Part model, mm, in its own coordinate system. Face numbers are marked on the shaded views. A direction names the side the tool comes from. Coordinates: 2 decimals unless noted, no trailing zeros. Write item = value, one per line. Start each with the question number.
Q1. Probe line 1 (Z direction, x = -103, y = -12.75); line 2 (Y direction, x = -108.5, z = -1.5). List the from-to ranges inside material, lowest first.
Q2. Pin check, flat tips, straight feed: P1, Ø6, axis at y = 6.5, z = 3.5, coming from the -X side; P2, Ø1.5, axis at x = -102.5, z = 9, coming from the +Y side; P3, Ø4, axis at x = -81, z = -5, coming from the -Y side. Stop position of each tip, or through.
Q3. Tool access for the marked faces 1, 2 and 3: list every direction of +Z, -Z, +X, -X, +Y, -Y with a clear straight run to the whole face (end or side of a thin tool).
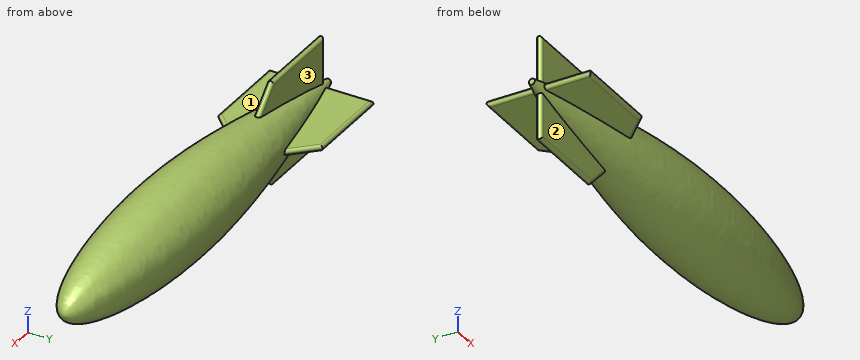
from build123d import *

# Parameters (mm, degrees)
CUT_EXTRUDE1_DEPTH      = 3.175
CUT_EXTRUDE1_DEPTH_BACK = 3.175
SKETCH3_R               = 6.509324081066561
BOSS_EXTRUDE5_DEPTH     = 0.79375
CIRPATTERN1_COUNT       = 4
FILLET2_R               = 0.79375


with BuildPart() as part:
    # Sketch2 → Revolve1 (revolve)
    with BuildSketch(Plane.XY):
        with BuildLine():
            Line((0, 0), (-127, -1.555e-14))
            add(Edge.make_bspline(
                [(-127, -1.555e-14), (-126.88600107696882, 0.01292807569490287), (-60.293650457458824, 18.501169159484686), (6.918e-14, 6.618926423252529), (0, 0)],
                knots=[0, 0, 0, 0, 0.5372544440165704, 1, 1, 1, 1], degree=3))
        make_face()
    revolve(axis=Axis((0, 0, 0), (-1, -1.2e-16, 0)))

    # Sketch3 → Cut-Extrude1 (cut, two sides: drawn at the far end of the back side and taken through both)
    with BuildSketch(Plane(origin=(-127, 0, 0), x_dir=(0, 0, -1), z_dir=(1, 0, 0)).offset(-CUT_EXTRUDE1_DEPTH_BACK)):
        Circle(SKETCH3_R)
    extrude(amount=CUT_EXTRUDE1_DEPTH + CUT_EXTRUDE1_DEPTH_BACK, mode=Mode.SUBTRACT)

    # Sketch4 → Boss-Extrude5 (add, symmetric)
    with BuildSketch(Plane.XY):
        Polygon((-120.64999999999937, 1.6175040904650868), (-120.65, 14.317504090465087), (-96.83750000000002, 14.317504090465087), (-90.2483075401766, 7.7283116306418425), (-89.68704153260985, 7.167045623074933), (-120.64999999999998, 0.8237540904650809), align=None)
    boss_extrude5 = extrude(amount=BOSS_EXTRUDE5_DEPTH, both=True)

    # CirPattern1: Boss-Extrude5 ×4 about axis
    cirpattern1_axis = Axis((0, -3.5e-16, 0), (1, 0, 0))
    for i in range(1, CIRPATTERN1_COUNT):
        add(boss_extrude5.rotate(cirpattern1_axis, i * 360 / CIRPATTERN1_COUNT))

    # Fillet2
    fillet2_edges = [part.edges().sort_by_distance(p)[0] for p in [
        (-93.52528303882053, 11.0052871292856, 0.79375),
        (-93.52528303882053, 11.005287129285604, -0.79375),
        (-108.74375, 14.317504090465087, -0.79375),
        (-108.74375, 14.317504090465087, 0.79375),
        (-120.64999999999999, 7.863429350843208, -0.79375),
        (-120.64999999999999, 7.863429350843208, 0.79375),
        (-120.64999999999999, 0.7937499999999978, -7.8634293508432105),
        (-120.64999999999999, -0.7937500000000021, -7.863429350843219),
        (-108.74375, 0.7937499999999964, -14.317504090465087),
        (-108.74375, -0.7937500000000035, -14.317504090465087),
        (-93.52528303882053, 0.7937499999999972, -11.005287129285605),
        (-93.52528303882053, -0.7937500000000027, -11.005287129285605),
        (-120.64999999999999, -7.863429350843224, -0.793749999999999),
        (-108.74375, -14.317504090465087, -0.7937499999999982),
        (-93.52528303882053, -11.005287129285612, -0.7937499999999986),
        (-120.64999999999999, -7.863429350843225, 0.793750000000001),
        (-93.52528303882053, -11.005287129285612, 0.7937500000000013),
        (-108.74375, -14.317504090465087, 0.7937500000000017),
        (-93.52528303882053, 0.7937500000000008, 11.005287129285605),
        (-93.52528303882053, -0.7937499999999991, 11.005287129285605),
        (-108.74375, -0.7937499999999987, 14.317504090465087),
        (-120.64999999999999, -0.7937499999999994, 7.8634293508432185),
        (-120.64999999999999, 0.7937500000000005, 7.863429350843211),
        (-108.74375, 0.7937500000000012, 14.317504090465087),
    ]]
    fillet(fillet2_edges, radius=FILLET2_R - 0.0001)  # a hair under: the kernel refuses the full size


solid = part.part
Ans:
q1.line_1 = -0.79 to 0.79
q1.line_2 = -4.1 to 4.1
q2.P1 = -120.47
q2.P2 = 0.79
q2.P3 = -8.61
q3.face_1 = +Z, -X, -Y
q3.face_2 = -Z, -X, -Y
q3.face_3 = +Z, -X, +Y
